```python
from build123d import *

# Parameters (mm, degrees)
SKETCH1_R            = 100
BOSS_EXTRUDE2_DEPTH  = 3
SKETCH5_W            = 3
SKETCH5_H            = 87
BOSS_EXTRUDE5_DEPTH  = 45
SKETCH8_W            = 3
SKETCH8_H            = 87
BOSS_EXTRUDE6_DEPTH  = 45
SKETCH9_W            = 23.719660605
SKETCH9_H            = 94.301811056
CUT_EXTRUDE2_DEPTH   = 45
SKETCH10_W           = 23.969699351
SKETCH10_H           = 92.447375273
CUT_EXTRUDE3_DEPTH   = 45
SKETCH11_R           = 6
CUT_EXTRUDE4_DEPTH   = 45
CUT_EXTRUDE5_START   = -45
SKETCH12_R           = 6
CUT_EXTRUDE5_DEPTH   = 45
BOSS_EXTRUDE7_DEPTH  = 45
CUT_EXTRUDE6_DEPTH   = 45
BOSS_EXTRUDE8_DEPTH  = 3
BOSS_EXTRUDE10_DEPTH = 3
SWEEP1_START         = 48
SWEEP1_DEPTH         = 300
BOSS_EXTRUDE11_START = -3
BOSS_EXTRUDE11_DEPTH = 3
SWEEP2_START         = -90
SWEEP2_DEPTH         = 180


# Read off the part's stored shape, not the designer's step: Sweep1, Sweep2
with BuildPart() as part:
    # Sketch1 → Boss-Extrude2 (new body)
    with BuildSketch(Plane(origin=(0, 0, 0), x_dir=(1, 0, 0), z_dir=(0, 1, 0))):
        with Locations(Location((0, 0, 0), (0, 0, 270))):
            Circle(SKETCH1_R)
    extrude(amount=BOSS_EXTRUDE2_DEPTH)

    # Sketch5 → Boss-Extrude5 (add)
    with BuildSketch(Plane(origin=(0, 3, 0), x_dir=(1, 0, 0), z_dir=(0, 1, 0))):
        with Locations((88.5, 0.088989435)):
            Rectangle(SKETCH5_W, SKETCH5_H)
    extrude(amount=BOSS_EXTRUDE5_DEPTH)

    # Sketch8 → Boss-Extrude6 (add)
    with BuildSketch(Plane(origin=(0, 3, 0), x_dir=(1, 0, 0), z_dir=(0, 1, 0))):
        with Locations((-88.5, 0.088989435)):
            Rectangle(SKETCH8_W, SKETCH8_H)
    extrude(amount=BOSS_EXTRUDE6_DEPTH)

    # Sketch9 → Cut-Extrude2 (cut)
    with BuildSketch(Plane(origin=(0, 3, 0), x_dir=(1, 0, 0), z_dir=(0, 1, 0))):
        with Locations((101.859830303, -3.561916093)):
            Rectangle(SKETCH9_W, SKETCH9_H)
    extrude(amount=-CUT_EXTRUDE2_DEPTH, mode=Mode.SUBTRACT)

    # Sketch10 → Cut-Extrude3 (cut)
    with BuildSketch(Plane(origin=(0, 3, 0), x_dir=(1, 0, 0), z_dir=(0, 1, 0))):
        with Locations((-101.984849676, 2.812677071)):
            Rectangle(SKETCH10_W, SKETCH10_H)
    extrude(amount=-CUT_EXTRUDE3_DEPTH, mode=Mode.SUBTRACT)

    # Sketch11 → Cut-Extrude4 (cut)
    with BuildSketch(Plane.ZY.offset(90)):
        with Locations((0, 33)):
            Circle(SKETCH11_R)
    extrude(amount=-CUT_EXTRUDE4_DEPTH, mode=Mode.SUBTRACT)

    # Sketch12 → Cut-Extrude5 (cut)
    with BuildSketch(Plane(origin=(90, 0, 0), x_dir=(0, 0, -1), z_dir=(1, 0, 0)).offset(CUT_EXTRUDE5_START)):
        with Locations(Location((0, 33, 0), (0, 0, 180))):
            Circle(SKETCH12_R)
    extrude(amount=CUT_EXTRUDE5_DEPTH, mode=Mode.SUBTRACT)

    # Sketch14 → Boss-Extrude7 (add)
    with BuildSketch(Plane(origin=(0, 3, 0), x_dir=(1, 0, 0), z_dir=(0, 1, 0))):
        with BuildLine():
            Line((-90, -43.411010565), (-90.085982049, -43.411010565))
            ThreePointArc((-90.085982049, -43.411010565), (-0.098829893, -99.999951163), (90, -43.588989435))
            Line((90, -43.588989435), (90, -43.411010565))
            Line((90, -43.411010565), (87, -43.411010565))
            Line((87, -43.411010565), (87, 43.588989435))
            Line((87, 43.588989435), (90, 43.588989435))
            ThreePointArc((90, 43.588989435), (0, 100), (-90, 43.588989435))
            Line((-90, 43.588989435), (-87, 43.588989435))
            Line((-87, 43.588989435), (-87, -43.411010565))
            Line((-87, -43.411010565), (-90, -43.411010565))
        make_face()
    extrude(amount=BOSS_EXTRUDE7_DEPTH)

    # 3DSketch1 → Cut-Extrude6 (cut)
    with BuildSketch(Plane(origin=(-87, 48, -42.895221179), x_dir=(0.8969072164948455, 0, 0.4422187750417981), z_dir=(0, -1, 0))):
        with BuildLine():
            Line((0, 0), (37.93814433, 76.946066857))
            ThreePointArc((37.93814433, 76.946066857), (139.895221179, 87), (194, 0))
            Line((194, 0), (156.06185567, -76.946066857))
            ThreePointArc((156.06185567, -76.946066857), (54.104778821, -87), (0, 0))
        make_face()
    extrude(amount=CUT_EXTRUDE6_DEPTH, mode=Mode.SUBTRACT)

    # Sketch17 → Boss-Extrude8 (add)
    with BuildSketch(Plane(origin=(90, 0, 0), x_dir=(0, 0, -1), z_dir=(1, 0, 0))):
        with BuildLine():
            Line((21.794494718, 348), (43.588989435, 348))
            Line((43.588989435, 348), (43.588989435, 48))
            Line((43.588989435, 48), (-43.588989435, 48))
            ThreePointArc((-43.588989435, 48), (11.635050375, 193.089199561), (21.794494718, 348))
        make_face()
    extrude(amount=-BOSS_EXTRUDE8_DEPTH)

    # Sketch21 → Boss-Extrude10 (add)
    with BuildSketch(Plane.ZY.offset(90)):
        with BuildLine():
            Line((43.411010565, 48), (-43.588989435, 48))
            Line((-43.588989435, 48), (-43.588989435, 348))
            Line((-43.588989435, 348), (-21.794494718, 348))
            ThreePointArc((-21.794494718, 348), (-11.721133915, 193.103198738), (43.411010565, 48))
        make_face()
    extrude(amount=-BOSS_EXTRUDE10_DEPTH)

    # Sweep1 outline → Sweep1 (add)
    with BuildSketch(Plane(origin=(0, 0, 0), x_dir=(1, 0, 0), z_dir=(0, 1, 0)).offset(SWEEP1_START)):
        with BuildLine():
            ThreePointArc((90, 43.588989435), (0, 100), (-90, 43.588989435))
            Line((-90, 43.588989435), (-87, 43.588989435))
            ThreePointArc((-87, 43.588989435), (0, 97.308786859), (87, 43.588989435))
            Line((87, 43.588989435), (90, 43.588989435))
        make_face()
    extrude(amount=SWEEP1_DEPTH)

    # Sketch26 → Boss-Extrude11 (add)
    with BuildSketch(Plane(origin=(0, 348, 0), x_dir=(1, 0, 0), z_dir=(0, 1, 0)).offset(BOSS_EXTRUDE11_START)):
        with BuildLine():
            Line((-90, 21.794494718), (90, 21.794494718))
            Line((90, 21.794494718), (90, 43.588989435))
            ThreePointArc((90, 43.588989435), (0, 100), (-90, 43.588989435))
            Line((-90, 43.588989435), (-90, 21.794494718))
        make_face()
    extrude(amount=BOSS_EXTRUDE11_DEPTH)

    # Sweep2 outline → Sweep2 (add)
    with BuildSketch(Plane.YZ.offset(SWEEP2_START)):
        with BuildLine():
            ThreePointArc((50.627921058, 41.94345394), (193.103198738, -11.721133915), (345, -22.038813222))
            Line((345, -22.038813222), (345, -21.794494718))
            ThreePointArc((345, -21.794494718), (191.70412896, -11.165627984), (48.136044185, 43.613947774))
            Line((48.136044185, 43.613947774), (50.627921058, 41.94345394))
        make_face()
    extrude(amount=SWEEP2_DEPTH)


solid = part.part
```
The listing builds one solid part. Answer for the finished solid, in the listing's coordinates (mm). A direction names the side the tool comes from. Coordinates: 2 decimals unless noted, no trailing zeros. Write each loop counter-clockwise with the first axis right and the second up, starting at its lowest first coordinate (ties: lowest second). Pieces come first, ordered by that corner, then holes. Notation, with made-up numbers: (69, 87.5) - (109, 87.5) arc R16 ccw to (109, 104.5) - close; hole circle Ø9 at (81.25, 66). An arc over 180 degrees is marked (long way). Return JSON: item names as keys, results as strings. Group by question number.
Q1. Which of the six approach directions +Z, -Z, +X, -X, +Y, -Y give full straight-line access (tool end or side, diameter ignored) to faces 5 (the cylindrical face through (-1.26, 193.814, -11.626)), 6 (the flat face through (-1, 345, -52))?
Q2. The part is cut by section D-D on z = -83. Write down the section's boundary in (x, y).
Q3. Flat-ended cylindrical pins translate along their axes: pin 1 Ø14 at (y, z) = (33, 0) entering from -X; pin 2 Ø10 at (x, z) = (0, 1.5) entering from -Y; pin 3 Ø5 at (x, z) = (69.5, -76.5) entering from +Y; pin 4 Ø0.9 at (x, y) = (19, 346.5) entering from +Z. Find the tip coordinate at first contact, or state that the pin passes through.
Q4. The part is cut by section B-B on z = 0. Write down the section's boundary in (x, y), and give its area (3 significant figures).
Q5. The part is cut by section C-C on x = -46. Write down the section's boundary in (y, z).
Q6. The part is cut by section A-A on y = 22. Write down the section's boundary in (x, z), and give its area (3 significant figures).
Q7. Find the intervals of material crossed by line 1 along X through (y, z) = (179, -39); line 2 along Y through (x, z) = (45.5, -36); line 3 along Y through (x, z) = (36, 62), in increasing order. Write a range as [from, to].
Q8. For a pull along X with two mould halves and no side action, classify faces 1 (the flat face through (1, 3, 2)), 2 (the flat face through (90, 133, -9)), 3 (the flat face through (-1, 348, -53)), 4 (the cylindrical face through (1.568, 171.564, -99.988)) as +X half, -X half, draft (parallel to the pull), parting line (faces both ways), or undercut.
Evaluation:
{
 "1": {"face 5": "+Z, +X, -X", "face 6": "none"},
 "2": {"outline": "(-55.78, 0) - (55.78, 0) - (55.78, 348) - (-55.78, 348) - close; hole (-50.79, 48) - (-50.2, 48) - (-50.2, 3) - (50.2, 3) - (50.2, 48) - (50.79, 48) - (50.79, 345) - (-50.79, 345) - close"},
 "3": {"pin 1": "stops at x = -90", "pin 2": "stops at y = 0", "pin 3": "passes through", "pin 4": "stops at z = -21.79"},
 "4": {"outline": "(-90, 0) - (90, 0) - (90, 27) - (87, 27) - (87, 3) - (-87, 3) - (-87, 27) - (-90, 27) - close; (-90, 39) - (-87, 39) - (-87, 148.68) - (87, 148.68) - (87, 39) - (90, 39) - (90, 149.51) - (-90, 149.51) - close", "area": "1,490 mm2"},
 "5": {"outline": "(0, -88.79) - (348, -88.79) - (348, -21.79) - (345, -21.79) arc R522.29 cw to (48.14, 43.61) - (50.63, 41.94) arc R522.53 ccw to (345, -22.04) - (345, -85.75) - (48, -85.75) - (48, -85.4) - (3, -85.4) - (3, 85.4) - (48, 85.4) - (48, 88.79) - (0, 88.79) - close"},
 "6": {"outline": "(-90.09, 43.41) - (-90, 43.41) - (-90, -43.59) arc R100 ccw to (90, -43.59) - (90, 43.59) arc R100 ccw to start; hole (-87, -42.9) arc R97 ccw to (87, -42.9) - (87, 42.9) arc R97 ccw to (-87, 42.9) - close", "area": "1,840 mm2"},
 "7": {"line 1": "x = [-90, -87], [87, 90]", "line 2": "y = [0, 3], [345, 348]", "line 3": "y = [0, 3]"},
 "8": {"face 1": "undercut", "face 2": "+X half", "face 3": "draft", "face 4": "parting line"}
}
